The model under review builds one solid part; all positions refer to its coordinate system, in mm. A direction names the side the tool comes from. Coordinates: 2 decimals unless noted, no trailing zeros. Loops run counter-clockwise (first coordinate to the right, second up) from the corner with the lowest first, then second, coordinate; pieces in that order, holes last. Notation, with made-up numbers: M 75,-12 L 91,-12 A12 cw 91,7 Z; hole C -3.5,33.25 d8. An arc over 180 degrees is marked long. Use one line per item in the form item = value.
```python
from build123d import *

# Parameters (mm, degrees)
F1_DEPTH     = 10.16
F2_T4_DEPTH  = 50.4313390776
F2_S5_R      = 6.4596874697
F2_T6_DEPTH  = 27
F2_T10_DEPTH = 50.4313390776
F2_S11_R     = 6.4596874697
F2_T12_DEPTH = 27
F2_T16_DEPTH = 50.4313390776
F2_S17_R     = 6.4596874697
F2_T18_DEPTH = 27
F2_T22_DEPTH = 50.4313390776
F2_S23_R     = 6.4596874697
F2_T24_DEPTH = 27
F3_T4_DEPTH  = 112.5049829483
F3_S5_R      = 6.4596874697
F3_T6_DEPTH  = 58
F3_T10_DEPTH = 112.5049829483
F3_S11_R     = 6.4596874697
F3_T12_DEPTH = 58
F3_T16_DEPTH = 112.5049829483
F3_S17_R     = 6.4596874697
F3_T18_DEPTH = 58
F3_T22_DEPTH = 112.5049829483
F3_S23_R     = 6.4596874697
F3_T24_DEPTH = 58


# Not quite as in the source:
# - a fillet or chamfer that OpenCascade refuses, or shapes differently, is made with other operations: its cross-section is extruded or revolved along the edge and cut away or added


with BuildPart() as f1:
    # F0 (on Front) → F1 (new body)
    with BuildSketch(Plane.XZ):
        with BuildLine():
            Line((-2.9818282316, 88.7313390776), (-2.9818282316, 50.8))
            ThreePointArc((-2.9818282316, 50.8), (-8.0369643669, 48.3618993886), (-9.2761479318, 42.8880378604))
            Line((-9.2761479318, 42.8880378604), (-9.2761479318, -44.6169450879))
            ThreePointArc((-9.2761479318, -44.6169450879), (-8.3117384594, -47.249729254), (-5.874895025, -48.6366078258))
            Line((-5.874895025, -48.6366078258), (0, -48.6366078258))
            Line((0, -48.6366078258), (5.874895025, -48.6366078258))
            ThreePointArc((5.874895025, -48.6366078258), (8.3117384594, -47.249729254), (9.2761479318, -44.6169450879))
            Line((9.2761479318, -44.6169450879), (9.2761479318, 42.8880378604))
            ThreePointArc((9.2761479318, 42.8880378604), (8.0369643669, 48.3618993886), (2.9818282316, 50.8))
            Line((2.9818282316, 50.8), (2.9818282316, 88.7313390776))
            Line((2.9818282316, 88.7313390776), (-2.9818282316, 88.7313390776))
        make_face()
    extrude(amount=F1_DEPTH)

    # F2: fillet of radius 2.5 on 4 edges, made by hand


with BuildPart() as f2_tool2:
    # F2_s3 → F2_t4 (new body)
    with BuildSketch(Plane.XY.offset(94.9813390776)):
        with BuildLine():
            ThreePointArc((-0.4818282316, 0), (-2.2495951845, -0.732233047), (-2.9818282316, -2.5))
            Line((-2.9818282316, -2.5), (-2.9818282316, 0))
            Line((-2.9818282316, 0), (-0.4818282316, 0))
        make_face()
    extrude(amount=-F2_T4_DEPTH)

    # F2_s5 → F2_t6 (cut, symmetric)
    with BuildSketch(Plane.XZ.offset(1.2)):
        with Locations((-2.9818282316, 44.3403125303)):
            Circle(F2_S5_R)
    extrude(amount=F2_T6_DEPTH, both=True, mode=Mode.SUBTRACT)


with BuildPart() as f1_1:
    add(f1.part)

    # F2_t1: cut F2_tool2
    add(f2_tool2.part, mode=Mode.SUBTRACT)


with BuildPart() as f2_tool8:
    # F2_s9 → F2_t10 (new body)
    with BuildSketch(Plane.XY.offset(44.55)):
        with BuildLine():
            ThreePointArc((0.4818282316, -10.16), (2.2495951845, -9.427766953), (2.9818282316, -7.66))
            Line((2.9818282316, -7.66), (2.9818282316, -10.16))
            Line((2.9818282316, -10.16), (0.4818282316, -10.16))
        make_face()
    extrude(amount=F2_T10_DEPTH)

    # F2_s11 → F2_t12 (cut, symmetric)
    with BuildSketch(Plane.XZ.offset(8.9)):
        with Locations((2.9818282316, 44.3403125303)):
            Circle(F2_S11_R)
    extrude(amount=F2_T12_DEPTH, both=True, mode=Mode.SUBTRACT)


with BuildPart() as f1_2:
    add(f1_1.part)

    # F2_t7: cut F2_tool8
    add(f2_tool8.part, mode=Mode.SUBTRACT)


with BuildPart() as f2_tool14:
    # F2_s15 → F2_t16 (new body)
    with BuildSketch(Plane.XY.offset(94.9813390776)):
        with BuildLine():
            ThreePointArc((-0.4818282316, -10.16), (-2.2495951845, -9.427766953), (-2.9818282316, -7.66))
            Line((-2.9818282316, -7.66), (-2.9818282316, -10.16))
            Line((-2.9818282316, -10.16), (-0.4818282316, -10.16))
        make_face()
    extrude(amount=-F2_T16_DEPTH)

    # F2_s17 → F2_t18 (cut, symmetric)
    with BuildSketch(Plane.XZ.offset(8.9)):
        with Locations((-2.9818282316, 44.3403125303)):
            Circle(F2_S17_R)
    extrude(amount=F2_T18_DEPTH, both=True, mode=Mode.SUBTRACT)


with BuildPart() as f1_3:
    add(f1_2.part)

    # F2_t13: cut F2_tool14
    add(f2_tool14.part, mode=Mode.SUBTRACT)


with BuildPart() as f2_tool20:
    # F2_s21 → F2_t22 (new body)
    with BuildSketch(Plane.XY.offset(44.55)):
        with BuildLine():
            ThreePointArc((0.4818282316, 0), (2.2495951845, -0.732233047), (2.9818282316, -2.5))
            Line((2.9818282316, -2.5), (2.9818282316, 0))
            Line((2.9818282316, 0), (0.4818282316, 0))
        make_face()
    extrude(amount=F2_T22_DEPTH)

    # F2_s23 → F2_t24 (cut, symmetric)
    with BuildSketch(Plane.XZ.offset(1.2)):
        with Locations((2.9818282316, 44.3403125303)):
            Circle(F2_S23_R)
    extrude(amount=F2_T24_DEPTH, both=True, mode=Mode.SUBTRACT)


with BuildPart() as f1_4:
    add(f1_3.part)

    # F2_t19: cut F2_tool20
    add(f2_tool20.part, mode=Mode.SUBTRACT)

    # F3: fillet of radius 5 on 4 edges, made by hand


with BuildPart() as f3_tool2:
    # F3_s3 → F3_t4 (new body)
    with BuildSketch(Plane.XY.offset(55.3880378604)):
        with BuildLine():
            ThreePointArc((-4.2761479318, 0), (-7.8116818377, -1.4644660941), (-9.2761479318, -5))
            Line((-9.2761479318, -5), (-9.2761479318, 0))
            Line((-9.2761479318, 0), (-4.2761479318, 0))
        make_face()
    extrude(amount=-F3_T4_DEPTH)

    # F3_s5 → F3_t6 (cut, symmetric)
    with BuildSketch(Plane.XZ.offset(2.5)):
        with Locations((-2.9818282316, 44.3403125303)):
            Circle(F3_S5_R)
    extrude(amount=F3_T6_DEPTH, both=True, mode=Mode.SUBTRACT)


with BuildPart() as f1_5:
    add(f1_4.part)

    # F3_t1: cut F3_tool2
    add(f3_tool2.part, mode=Mode.SUBTRACT)


with BuildPart() as f3_tool8:
    # F3_s9 → F3_t10 (new body)
    with BuildSketch(Plane.XY.offset(-57.1169450879)):
        with BuildLine():
            ThreePointArc((4.2761479318, 0), (7.8116818377, -1.4644660941), (9.2761479318, -5))
            Line((9.2761479318, -5), (9.2761479318, 0))
            Line((9.2761479318, 0), (4.2761479318, 0))
        make_face()
    extrude(amount=F3_T10_DEPTH)

    # F3_s11 → F3_t12 (cut, symmetric)
    with BuildSketch(Plane.XZ.offset(2.5)):
        with Locations((2.9818282316, 44.3403125303)):
            Circle(F3_S11_R)
    extrude(amount=F3_T12_DEPTH, both=True, mode=Mode.SUBTRACT)


with BuildPart() as f1_6:
    add(f1_5.part)

    # F3_t7: cut F3_tool8
    add(f3_tool8.part, mode=Mode.SUBTRACT)


with BuildPart() as f3_tool14:
    # F3_s15 → F3_t16 (new body)
    with BuildSketch(Plane.XY.offset(55.3880378604)):
        with BuildLine():
            ThreePointArc((-4.2761479318, -10.16), (-7.8116818377, -8.6955339059), (-9.2761479318, -5.16))
            Line((-9.2761479318, -5.16), (-9.2761479318, -10.16))
            Line((-9.2761479318, -10.16), (-4.2761479318, -10.16))
        make_face()
    extrude(amount=-F3_T16_DEPTH)

    # F3_s17 → F3_t18 (cut, symmetric)
    with BuildSketch(Plane.XZ.offset(7.7)):
        with Locations((-2.9818282316, 44.3403125303)):
            Circle(F3_S17_R)
    extrude(amount=F3_T18_DEPTH, both=True, mode=Mode.SUBTRACT)


with BuildPart() as f1_7:
    add(f1_6.part)

    # F3_t13: cut F3_tool14
    add(f3_tool14.part, mode=Mode.SUBTRACT)


with BuildPart() as f3_tool20:
    # F3_s21 → F3_t22 (new body)
    with BuildSketch(Plane.XY.offset(-57.1169450879)):
        with BuildLine():
            ThreePointArc((4.2761479318, -10.16), (7.8116818377, -8.6955339059), (9.2761479318, -5.16))
            Line((9.2761479318, -5.16), (9.2761479318, -10.16))
            Line((9.2761479318, -10.16), (4.2761479318, -10.16))
        make_face()
    extrude(amount=F3_T22_DEPTH)

    # F3_s23 → F3_t24 (cut, symmetric)
    with BuildSketch(Plane.XZ.offset(7.7)):
        with Locations((2.9818282316, 44.3403125303)):
            Circle(F3_S23_R)
    extrude(amount=F3_T24_DEPTH, both=True, mode=Mode.SUBTRACT)


with BuildPart() as f1_8:
    add(f1_7.part)

    # F3_t19: cut F3_tool20
    add(f3_tool20.part, mode=Mode.SUBTRACT)


solid = f1_8.part
```
1. Wall thickness on line 1 along X through (y, z) = (-7, 73.5); line 2 along Z through (x, y) = (-3.5, -3); line 3 along X through (y, z) = (-5.5, -27): over which ranges is each line inside the solid? List them lowest first. Write a range as from..to.
Response values:
line_1 = -2.98..2.98
line_2 = -48.64..50.78
line_3 = -9.26..9.26
2. Insertion check: P1, Ø1, axis at x = 2.5, z = 69, coming from the +Y side; P2, Ø4, axis at y = -5, z = 78, coming from the -X side; P3, Ø4, axis at y = -5.5, z = 62, coming from the +X side. Each pin has a flat end and moves straight along its axis. Give the tip position at first contact, or say it passes through.
Response values:
P1 = -0.51
P2 = -2.98
P3 = 2.98
3. Add section A-A (z = 76). State the section outline as (x, y) points, then the cut area to 3 significant figures.
Response values:
outline = M -2.98,-7.66 A2.5 ccw -0.48,-10.16 L 0.48,-10.16 A2.5 ccw 2.98,-7.66 L 2.98,-2.5 A2.5 ccw 0.48,0 L -0.48,0 A2.5 ccw -2.98,-2.5 Z
area = 55.2 mm^2
4. Add section B-B (y = -3.75). State the section outline as (x, z) points.
Response values:
outline = M -9.12,-45.74 A4.08 ccw -5.87,-48.64 L 5.87,-48.64 A4.08 ccw 9.12,-45.74 L 9.12,42.32 A6.46 ccw 2.98,50.8 L 2.98,88.73 L -2.98,88.73 L -2.98,50.8 A6.46 ccw -9.12,42.32 Z
5. Machinability: for faces 1 (the face through (2.982, -5, 70)), 2 (the face through (7.773, -8.734, -3.515)), 3 (the face through (-7.773, -8.734, -2.234)), 4 (the face through (-2.982, -5, 70)), which of the approach directions +Z, -Z, +X, -X, +Y, -Y give a long, thin tool a straight path to every point of the face, cutting with its end or side? Answer none if there is none.
Response values:
face_1 = +Z, +X, +Y, -Y
face_2 = -Z, +X, -Y
face_3 = -Z, -X, -Y
face_4 = +Z, -X, +Y, -Y
6. Add section C-C (x = 7). State the section outline as (y, z) points.
Response values:
outline = M -10.16,39.28 L -9.35,39.28 L -9.35,-48.27 L -0.81,-48.27 L -0.81,39.28 L 0,39.28 L 0,49.4 L -10.16,49.4 Z
7. Add section D-D (z = 25). State the section outline as (x, y) points, then the cut area to 3 significant figures.
Response values:
outline = M -9.28,-5.16 A5 ccw -4.28,-10.16 L 4.28,-10.16 A5 ccw 9.28,-5.16 L 9.28,-5 A5 ccw 4.28,0 L -4.28,0 A5 ccw -9.28,-5 Z
area = 167 mm^2
